For this review, take the finished solid that the model builds, in its own axes (mm). Face numbers are marked on the shaded views. A direction names the side the tool comes from. Coordinates: 2 decimals unless noted, no trailing zeros. Order: outer loops, then holes, each group sorted by start corner. A loop starts at its lowest first (then second) coordinate and runs counter-clockwise, first axis right, second up. Notation, with made-up numbers: (48, -23.5) -> (73, -23.5) arc R14 cw to (73, -10.5) -> close; hole circle Ø4 at (19.25, -16.75). An arc over 180 degrees is marked (long way). Write item = value, one per line. Start each with the question number.
1) Consider section A-A on y = 0. Give the boundary of the cut face in (x, z), and give its area (3 significant figures).
2) Consider section B-B on z = 35. Give the boundary of the cut face in (x, y).
3) Wall thickness on probe 1 along Y at (x, z) = (-13, 5.5); probe 2 along Y at (x, z) = (-7.5, 34.5); probe 3 along X at (y, z) = (47.5, 33): over which ranges is each line inside the solid? List them lowest first. Write a range as [from, to].
4) Insertion check: pin 1 Ø5 at (x, z) = (-1, 22) entering from -Y; pin 2 Ø8 at (x, y) = (10.72, -41.54) entering from +Z; pin 3 Ø24 at (x, z) = (8.5, 30.5) entering from -Y; pin 4 Ø8 at (x, y) = (5, -14.5) entering from +Z. Each pin has a flat end and moves straight along its axis. Give the tip position at first contact, or say it passes through.
5) Consider section D-D on z = 21.5. Give the boundary of the cut face in (x, y).
6) Machinability: for the marked faces 5, 6, 7 and 8, which of the approach directions +Z, -Z, +X, -X, +Y, -Y give a long, thin tool a straight path to every point of the face, cutting with its end or side? Answer none if there is none.
7) Draft analysis for pull direction Y (two halves, no side actions). For the marked faces 1, 2, 3 and 4, state which applies: +Y half, -Y half, draft (parallel to the pull), parting line (faces both ways), or undercut.
8) Consider section C-C on x = 11. Give the boundary of the cut face in (y, z).
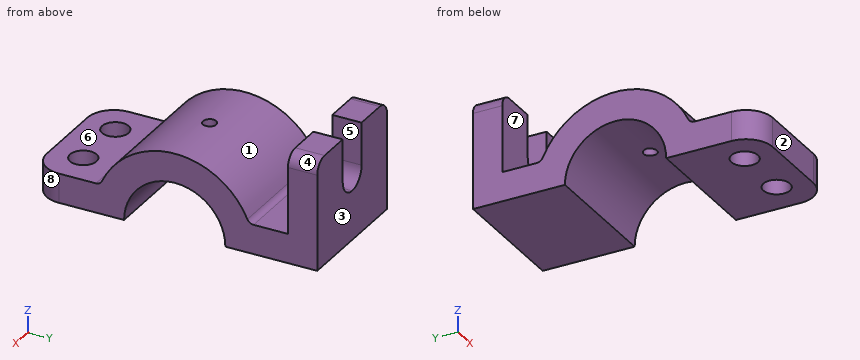
from build123d import *

# Parameters (mm, degrees)
F1_DEPTH  = 24
F2_R      = 5
F3_R      = 5
F5_DEPTH  = 25.4
F7_R      = 2.54
F6_R      = 2.5
F8_DEPTH  = 25.4
F10_R     = 10
F9_R      = 5
F11_DEPTH = 25.4


with BuildPart() as f1:
    # F0 (on Right) → F1 (new body, symmetric)
    with BuildSketch(Plane.YZ):
        with BuildLine():
            ThreePointArc((-30, 0), (-29.4730143031, 5.5983415304), (-27.9105714739, 11))
            Line((-27.9105714739, 11), (-53.5, 11))
            Line((-53.5, 11), (-53.5, 0))
            Line((-53.5, 0), (-30, 0))
        make_face()
        with BuildLine():
            Line((-15.4919333848, 11), (-27.9105714739, 11))
            ThreePointArc((-27.9105714739, 11), (-29.4730143031, 5.5983415304), (-30, 0))
            Line((-30, 0), (-19, 0))
            ThreePointArc((-19, 0), (-18.1017503893, 5.7729223833), (-15.4919333848, 11))
        make_face()
        with BuildLine():
            Line((15.4919333848, 11), (27.9105714739, 11))
            ThreePointArc((27.9105714739, 11), (0, 30), (-27.9105714739, 11))
            Line((-27.9105714739, 11), (-15.4919333848, 11))
            ThreePointArc((-15.4919333848, 11), (0, 19), (15.4919333848, 11))
        make_face()
        with BuildLine():
            Line((19, 0), (30, 0))
            ThreePointArc((30, 0), (29.4730143031, 5.5983415304), (27.9105714739, 11))
            Line((27.9105714739, 11), (15.4919333848, 11))
            ThreePointArc((15.4919333848, 11), (18.1017503893, 5.7729223833), (19, 0))
        make_face()
        with BuildLine():
            Line((30, 0), (42.5, 0))
            Line((42.5, 0), (42.5, 11))
            Line((42.5, 11), (27.9105714739, 11))
            ThreePointArc((27.9105714739, 11), (29.4730143031, 5.5983415304), (30, 0))
        make_face()
        Polygon((42.5, 0), (53.5, 0), (53.5, 41), (42.5, 41), (42.5, 11), align=None)
    extrude(amount=F1_DEPTH, both=True)

    # F2
    f2_edges = [f1.edges().sort_by_distance(p)[0] for p in [
        (24, 48, 41),
    ]]
    fillet(f2_edges, radius=F2_R)

    # F3
    f3_edges = [f1.edges().sort_by_distance(p)[0] for p in [
        (-24, 48, 41),
    ]]
    fillet(f3_edges, radius=F3_R)

    # F4 (on face) → F5 (cut)
    with BuildSketch(Plane(origin=(0, 53.5, 0), x_dir=(-1, 0, 0), z_dir=(0, 1, 0))):
        with BuildLine():
            ThreePointArc((6.5, 25), (0, 31.5), (-6.5, 25))
            ThreePointArc((-6.5, 25), (-4.5961940777, 20.4038059223), (0, 18.5))
            ThreePointArc((0, 18.5), (4.5961940777, 20.4038059223), (6.5, 25))
        make_face()
        with BuildLine():
            Line((6.5, 41), (-6.5, 41))
            Line((-6.5, 41), (-6.5, 25))
            ThreePointArc((-6.5, 25), (0, 31.5), (6.5, 25))
            Line((6.5, 25), (6.5, 41))
        make_face()
    extrude(amount=-F5_DEPTH, mode=Mode.SUBTRACT)

    # F7
    f7_edges = [f1.edges().sort_by_distance(p)[0] for p in [
        (0, 27.910571, 11),
        (0, -27.910571, 11),
    ]]
    fillet(f7_edges, radius=F7_R)

    # F6 (on face) → F8 (cut)
    with BuildSketch(Plane.XY.offset(11)):
        Circle(F6_R)
    extrude(amount=F8_DEPTH, mode=Mode.SUBTRACT)

    # F10
    f10_edges = [f1.edges().sort_by_distance(p)[0] for p in [
        (-24, -53.5, 5.5),
        (24, -53.5, 5.5),
    ]]
    fillet(f10_edges, radius=F10_R)

    # F9 (on face) → F11 (cut)
    with BuildSketch(Plane.XY.offset(11)):
        with Locations((-11.3169830292, -41.5445936071)):
            Circle(F9_R)
        with Locations((10.7156652957, -41.5445936071)):
            Circle(F9_R)
    extrude(amount=-F11_DEPTH, mode=Mode.SUBTRACT)


solid = f1.part
Answer sheet:
q1.outline = (-24, 19) -> (-2.5, 19) -> (-2.5, 30) -> (-24, 30) -> close; (2.5, 19) -> (24, 19) -> (24, 30) -> (2.5, 30) -> close
q1.area = 473 mm2
q2.outline = (-24, 42.5) -> (-6.5, 42.5) -> (-6.5, 53.5) -> (-24, 53.5) -> close; (6.5, 42.5) -> (24, 42.5) -> (24, 53.5) -> (6.5, 53.5) -> close
q3.probe_1 = [-53.5, -46.25], [-36.84, -18.19], [18.19, 53.5]
q3.probe_2 = [42.5, 53.5]
q3.probe_3 = [-24, -6.5], [6.5, 24]
q4.pin_1 = -22.8
q4.pin_2 = through
q4.pin_3 = -23.62
q4.pin_4 = 28.1
q5.outline = (-24, -20.92) -> (24, -20.92) -> (24, 20.92) -> (-24, 20.92) -> close; (-24, 42.5) -> (-5.48, 42.5) -> (-5.48, 53.5) -> (-24, 53.5) -> close; (5.48, 42.5) -> (24, 42.5) -> (24, 53.5) -> (5.48, 53.5) -> close; hole circle Ø5 at (0, 0)
q6.face_5 = +Z, +Y
q6.face_6 = +Z, +X, -X, -Y
q6.face_7 = +Z, +X, -X
q6.face_8 = +Z, -Z, +X, -Y
q7.face_1 = undercut
q7.face_2 = -Y half
q7.face_3 = +Y half
q7.face_4 = draft
q8.outline = (-53.5, 0) -> (-46.54, 0) -> (-46.54, 11) -> (-53.5, 11) -> close; (-36.55, 0) -> (-19, 0) arc R19 cw to (19, 0) -> (53.5, 0) -> (53.5, 41) -> (42.5, 41) -> (42.5, 11) -> (29.59, 11) arc R2.54 cw to (27.28, 12.48) arc R30 ccw to (-27.28, 12.48) arc R2.54 cw to (-29.59, 11) -> (-36.55, 11) -> close
